```python
from build123d import *

# Parameters (mm, degrees)
BOSS_EXTRU_1_DEPTH       = 15
ESQUISSE6_W              = 100
ESQUISSE6_H              = 15
ENL_V_MAT_EXTRU_1_DEPTH  = 255
ENL_V_MAT_EXTRU_10_REACH = 393.106
ESQUISSE11_R             = 2.25
ENL_V_MAT_EXTRU_11_REACH = 393.106
ESQUISSE8_R              = 2.25
CONG_10_R                = 10
CONG_11_R                = 2
ENL_V_MAT_EXTRU_12_REACH = 391.991
ENL_V_MAT_EXTRU_13_REACH = 391.991
ESQUISSE13_W             = 20
ESQUISSE13_H             = 143.033455182
ESQUISSE13_H_2           = 181.308681646
CONG_12_R                = 10
ENL_V_MAT_EXTRU_14_REACH = 376.645
ESQUISSE14_R             = 1.6


with BuildPart() as part:
    # Esquisse1 → Boss.-Extru.1 (new body)
    with BuildSketch(Plane(origin=(0, 0, 0), x_dir=(1, 0, 0), z_dir=(0, 1, 0))):
        Polygon((-76.643189126, -51.401333399), (63.356810874, 43.598666601), (163.356810874, 43.598666601), (303.356810874, -51.401333399), (303.356810874, -151.401333399), (163.356810874, -246.401333399), (63.356810874, -246.401333399), (-76.643189126, -151.401333399), align=None)
    extrude(amount=BOSS_EXTRU_1_DEPTH)

    # Esquisse6 → Enlèv. mat.-Extru.1 (cut)
    with BuildSketch(Plane.XY.offset(246.401333399)):
        with Locations((113.356810874, 7.5)):
            Rectangle(ESQUISSE6_W, ESQUISSE6_H)
    extrude(amount=-ENL_V_MAT_EXTRU_1_DEPTH, mode=Mode.SUBTRACT)

    # Esquisse11 → Enlèv. mat.-Extru.10 (cut, up to next)
    with BuildSketch(Plane(origin=(0, 15, 0), x_dir=(1, 0, 0), z_dir=(0, 1, 0)), mode=Mode.PRIVATE) as enl_v_mat_extru_10_sk1:
        with Locations(Location((53.356810874, -129.901333399, 0), (0, 0, 270))):
            Circle(ESQUISSE11_R)
    enl_v_mat_extru_10_tool1 = extrude(enl_v_mat_extru_10_sk1.sketch, amount=-ENL_V_MAT_EXTRU_10_REACH, mode=Mode.PRIVATE) & part.part
    # Esquisse11 → Enlèv. mat.-Extru.10 (cut, up to next)
    with BuildSketch(Plane(origin=(0, 15, 0), x_dir=(1, 0, 0), z_dir=(0, 1, 0)), mode=Mode.PRIVATE) as enl_v_mat_extru_10_sk2:
        with Locations(Location((53.356810874, -184.901333399, 0), (0, 0, 270))):
            Circle(ESQUISSE11_R)
    enl_v_mat_extru_10_tool2 = extrude(enl_v_mat_extru_10_sk2.sketch, amount=-ENL_V_MAT_EXTRU_10_REACH, mode=Mode.PRIVATE) & part.part
    # Esquisse11 → Enlèv. mat.-Extru.10 (cut, up to next)
    with BuildSketch(Plane(origin=(0, 15, 0), x_dir=(1, 0, 0), z_dir=(0, 1, 0)), mode=Mode.PRIVATE) as enl_v_mat_extru_10_sk3:
        with Locations(Location((173.356810874, -129.901333399, 0), (0, 0, 270))):
            Circle(ESQUISSE11_R)
    enl_v_mat_extru_10_tool3 = extrude(enl_v_mat_extru_10_sk3.sketch, amount=-ENL_V_MAT_EXTRU_10_REACH, mode=Mode.PRIVATE) & part.part
    # Esquisse11 → Enlèv. mat.-Extru.10 (cut, up to next)
    with BuildSketch(Plane(origin=(0, 15, 0), x_dir=(1, 0, 0), z_dir=(0, 1, 0)), mode=Mode.PRIVATE) as enl_v_mat_extru_10_sk4:
        with Locations(Location((173.356810874, -184.901333399, 0), (0, 0, 270))):
            Circle(ESQUISSE11_R)
    enl_v_mat_extru_10_tool4 = extrude(enl_v_mat_extru_10_sk4.sketch, amount=-ENL_V_MAT_EXTRU_10_REACH, mode=Mode.PRIVATE) & part.part
    add(enl_v_mat_extru_10_tool1.solids().sort_by_distance((53.356811, 15, 129.901333))[0], mode=Mode.SUBTRACT)
    add(enl_v_mat_extru_10_tool2.solids().sort_by_distance((53.356811, 15, 184.901333))[0], mode=Mode.SUBTRACT)
    add(enl_v_mat_extru_10_tool3.solids().sort_by_distance((173.356811, 15, 129.901333))[0], mode=Mode.SUBTRACT)
    add(enl_v_mat_extru_10_tool4.solids().sort_by_distance((173.356811, 15, 184.901333))[0], mode=Mode.SUBTRACT)

    # Esquisse8 → Enlèv. mat.-Extru.11 (cut, up to next)
    with BuildSketch(Plane(origin=(0, 15, 0), x_dir=(1, 0, 0), z_dir=(0, 1, 0)), mode=Mode.PRIVATE) as enl_v_mat_extru_11_sk1:
        with Locations(Location((180.356810874, -120.901333399, 0), (0, 0, 270))):
            Circle(ESQUISSE8_R)
    enl_v_mat_extru_11_tool1 = extrude(enl_v_mat_extru_11_sk1.sketch, amount=-ENL_V_MAT_EXTRU_11_REACH, mode=Mode.PRIVATE) & part.part
    # Esquisse8 → Enlèv. mat.-Extru.11 (cut, up to next)
    with BuildSketch(Plane(origin=(0, 15, 0), x_dir=(1, 0, 0), z_dir=(0, 1, 0)), mode=Mode.PRIVATE) as enl_v_mat_extru_11_sk2:
        with Locations(Location((180.356810874, -81.901333399, 0), (0, 0, 270))):
            Circle(ESQUISSE8_R)
    enl_v_mat_extru_11_tool2 = extrude(enl_v_mat_extru_11_sk2.sketch, amount=-ENL_V_MAT_EXTRU_11_REACH, mode=Mode.PRIVATE) & part.part
    # Esquisse8 → Enlèv. mat.-Extru.11 (cut, up to next)
    with BuildSketch(Plane(origin=(0, 15, 0), x_dir=(1, 0, 0), z_dir=(0, 1, 0)), mode=Mode.PRIVATE) as enl_v_mat_extru_11_sk3:
        with Locations(Location((46.356810874, -120.901333399, 0), (0, 0, 270))):
            Circle(ESQUISSE8_R)
    enl_v_mat_extru_11_tool3 = extrude(enl_v_mat_extru_11_sk3.sketch, amount=-ENL_V_MAT_EXTRU_11_REACH, mode=Mode.PRIVATE) & part.part
    # Esquisse8 → Enlèv. mat.-Extru.11 (cut, up to next)
    with BuildSketch(Plane(origin=(0, 15, 0), x_dir=(1, 0, 0), z_dir=(0, 1, 0)), mode=Mode.PRIVATE) as enl_v_mat_extru_11_sk4:
        with Locations(Location((46.356810874, -81.901333399, 0), (0, 0, 270))):
            Circle(ESQUISSE8_R)
    enl_v_mat_extru_11_tool4 = extrude(enl_v_mat_extru_11_sk4.sketch, amount=-ENL_V_MAT_EXTRU_11_REACH, mode=Mode.PRIVATE) & part.part
    add(enl_v_mat_extru_11_tool1.solids().sort_by_distance((180.356811, 15, 120.901333))[0], mode=Mode.SUBTRACT)
    add(enl_v_mat_extru_11_tool2.solids().sort_by_distance((180.356811, 15, 81.901333))[0], mode=Mode.SUBTRACT)
    add(enl_v_mat_extru_11_tool3.solids().sort_by_distance((46.356811, 15, 120.901333))[0], mode=Mode.SUBTRACT)
    add(enl_v_mat_extru_11_tool4.solids().sort_by_distance((46.356811, 15, 81.901333))[0], mode=Mode.SUBTRACT)

    # Congé10
    cong_10_edges = [part.edges().sort_by_distance(p)[0] for p in [
        (-76.643189126, 7.5, 51.401333399),
        (63.356810874, 7.5, -43.598666601),
        (163.356810874, 7.5, -43.598666601),
        (303.356810874, 7.5, 51.401333399),
        (303.356810874, 7.5, 151.401333399),
        (-76.643189126, 7.5, 151.401333399),
        (63.356810874, 7.5, -8.598666601),
        (163.356810874, 7.5, -8.598666601),
    ]]
    fillet(cong_10_edges, radius=CONG_10_R)

    # Congé11
    cong_11_edges = [part.edges().sort_by_distance(p)[0] for p in [
        (163.356810874, 7.5, 246.401333399),
        (63.356810874, 7.5, 246.401333399),
    ]]
    fillet(cong_11_edges, radius=CONG_11_R)

    # Esquisse12 → Enlèv. mat.-Extru.12 (cut, up to next)
    with BuildSketch(Plane(origin=(0, 15, 0), x_dir=(1, 0, 0), z_dir=(0, 1, 0)), mode=Mode.PRIVATE) as enl_v_mat_extru_12_sk1:
        with BuildLine():
            Line((34.940182765, -48.918575783), (15.793326272, -80.935246354))
            ThreePointArc((15.793326272, -80.935246354), (14.39255048, -85.48771654), (15.256670784, -90.171780344))
            Line((15.256670784, -90.171780344), (27.943631129, -118.361875593))
            ThreePointArc((27.943631129, -118.361875593), (31.633138728, -122.655474578), (37.06267458, -124.257847507))
            Line((37.06267458, -124.257847507), (53.356810874, -124.257847507))
            ThreePointArc((53.356810874, -124.257847507), (57.183645198, -123.496642832), (60.427878686, -121.328915318))
            Line((60.427878686, -121.328915318), (63.356810874, -118.39998313))
            Line((63.356810874, -118.39998313), (63.356810874, -59.592280682))
            Line((63.356810874, -59.592280682), (64.824779414, -43.572926285))
            ThreePointArc((64.824779414, -43.572926285), (48.973323725, -41.163150472), (34.940182765, -48.918575783))
        make_face()
    enl_v_mat_extru_12_tool1 = extrude(enl_v_mat_extru_12_sk1.sketch, amount=-ENL_V_MAT_EXTRU_12_REACH, mode=Mode.PRIVATE) & part.part
    # Esquisse12 → Enlèv. mat.-Extru.12 (cut, up to next)
    with BuildSketch(Plane(origin=(0, 15, 0), x_dir=(1, 0, 0), z_dir=(0, 1, 0)), mode=Mode.PRIVATE) as enl_v_mat_extru_12_sk2:
        with BuildLine():
            Line((166.285743062, -121.328915318), (163.356810874, -118.39998313))
            Line((163.356810874, -118.39998313), (163.356810874, -73.642376596))
            Line((163.356810874, -73.642376596), (176.462200108, -67.250451181))
            ThreePointArc((176.462200108, -67.250451181), (187.921289626, -66.549583242), (196.519678004, -74.156794674))
            Line((196.519678004, -74.156794674), (206.924784537, -95.490424571))
            ThreePointArc((206.924784537, -95.490424571), (205.909865534, -114.856232791), (188.948903611, -124.257847507))
            Line((188.948903611, -124.257847507), (173.356810874, -124.257847507))
            ThreePointArc((173.356810874, -124.257847507), (169.529976551, -123.496642832), (166.285743062, -121.328915318))
        make_face()
    enl_v_mat_extru_12_tool2 = extrude(enl_v_mat_extru_12_sk2.sketch, amount=-ENL_V_MAT_EXTRU_12_REACH, mode=Mode.PRIVATE) & part.part
    add(enl_v_mat_extru_12_tool1.solids().sort_by_distance((43.224361, 15, 84.406415))[0], mode=Mode.SUBTRACT)
    add(enl_v_mat_extru_12_tool2.solids().sort_by_distance((183.873626, 15, 97.045657))[0], mode=Mode.SUBTRACT)

    # Esquisse13 → Enlèv. mat.-Extru.13 (cut, up to next)
    with BuildSketch(Plane(origin=(0, 15, 0), x_dir=(1, 0, 0), z_dir=(0, 1, 0)), mode=Mode.PRIVATE) as enl_v_mat_extru_13_sk1:
        with Locations((-66.643189126, -101.968599131)):
            Rectangle(ESQUISSE13_W, ESQUISSE13_H)
    enl_v_mat_extru_13_tool1 = extrude(enl_v_mat_extru_13_sk1.sketch, amount=-ENL_V_MAT_EXTRU_13_REACH, mode=Mode.PRIVATE) & part.part
    # Esquisse13 → Enlèv. mat.-Extru.13 (cut, up to next)
    with BuildSketch(Plane(origin=(0, 15, 0), x_dir=(1, 0, 0), z_dir=(0, 1, 0)), mode=Mode.PRIVATE) as enl_v_mat_extru_13_sk2:
        with Locations((293.356810874, -101.059068944)):
            Rectangle(ESQUISSE13_W, ESQUISSE13_H_2)
    enl_v_mat_extru_13_tool2 = extrude(enl_v_mat_extru_13_sk2.sketch, amount=-ENL_V_MAT_EXTRU_13_REACH, mode=Mode.PRIVATE) & part.part
    add(enl_v_mat_extru_13_tool1.solids().sort_by_distance((-66.643189, 15, 101.968599))[0], mode=Mode.SUBTRACT)
    add(enl_v_mat_extru_13_tool2.solids().sort_by_distance((293.356811, 15, 101.059069))[0], mode=Mode.SUBTRACT)

    # Congé12
    cong_12_edges = [part.edges().sort_by_distance(p)[0] for p in [
        (-56.643189126, 7.5, 37.829904828),
        (-56.643189126, 7.5, 164.97276197),
        (283.356810874, 7.5, 37.829904828),
        (283.356810874, 7.5, 164.97276197),
    ]]
    fillet(cong_12_edges, radius=CONG_12_R)

    # Esquisse14 → Enlèv. mat.-Extru.14 (cut, up to next)
    with BuildSketch(Plane(origin=(0, 15, 0), x_dir=(1, 0, 0), z_dir=(0, 1, 0)), mode=Mode.PRIVATE) as enl_v_mat_extru_14_sk1:
        with Locations(Location((-42.643189126, -51.403530316, 0), (0, 0, 270))):
            Circle(ESQUISSE14_R)
    enl_v_mat_extru_14_tool1 = extrude(enl_v_mat_extru_14_sk1.sketch, amount=-ENL_V_MAT_EXTRU_14_REACH, mode=Mode.PRIVATE) & part.part
    # Esquisse14 → Enlèv. mat.-Extru.14 (cut, up to next)
    with BuildSketch(Plane(origin=(0, 15, 0), x_dir=(1, 0, 0), z_dir=(0, 1, 0)), mode=Mode.PRIVATE) as enl_v_mat_extru_14_sk2:
        with Locations(Location((-42.643189126, -151.403530316, 0), (0, 0, 270))):
            Circle(ESQUISSE14_R)
    enl_v_mat_extru_14_tool2 = extrude(enl_v_mat_extru_14_sk2.sketch, amount=-ENL_V_MAT_EXTRU_14_REACH, mode=Mode.PRIVATE) & part.part
    # Esquisse14 → Enlèv. mat.-Extru.14 (cut, up to next)
    with BuildSketch(Plane(origin=(0, 15, 0), x_dir=(1, 0, 0), z_dir=(0, 1, 0)), mode=Mode.PRIVATE) as enl_v_mat_extru_14_sk3:
        with Locations(Location((73.359258963, 29.598666601, 0), (0, 0, 270))):
            Circle(ESQUISSE14_R)
    enl_v_mat_extru_14_tool3 = extrude(enl_v_mat_extru_14_sk3.sketch, amount=-ENL_V_MAT_EXTRU_14_REACH, mode=Mode.PRIVATE) & part.part
    # Esquisse14 → Enlèv. mat.-Extru.14 (cut, up to next)
    with BuildSketch(Plane(origin=(0, 15, 0), x_dir=(1, 0, 0), z_dir=(0, 1, 0)), mode=Mode.PRIVATE) as enl_v_mat_extru_14_sk4:
        with Locations(Location((153.359258963, 29.598666601, 0), (0, 0, 270))):
            Circle(ESQUISSE14_R)
    enl_v_mat_extru_14_tool4 = extrude(enl_v_mat_extru_14_sk4.sketch, amount=-ENL_V_MAT_EXTRU_14_REACH, mode=Mode.PRIVATE) & part.part
    # Esquisse14 → Enlèv. mat.-Extru.14 (cut, up to next)
    with BuildSketch(Plane(origin=(0, 15, 0), x_dir=(1, 0, 0), z_dir=(0, 1, 0)), mode=Mode.PRIVATE) as enl_v_mat_extru_14_sk5:
        with Locations(Location((269.356810874, -51.399136482, 0), (0, 0, 270))):
            Circle(ESQUISSE14_R)
    enl_v_mat_extru_14_tool5 = extrude(enl_v_mat_extru_14_sk5.sketch, amount=-ENL_V_MAT_EXTRU_14_REACH, mode=Mode.PRIVATE) & part.part
    # Esquisse14 → Enlèv. mat.-Extru.14 (cut, up to next)
    with BuildSketch(Plane(origin=(0, 15, 0), x_dir=(1, 0, 0), z_dir=(0, 1, 0)), mode=Mode.PRIVATE) as enl_v_mat_extru_14_sk6:
        with Locations(Location((269.356810874, -141.399136482, 0), (0, 0, 270))):
            Circle(ESQUISSE14_R)
    enl_v_mat_extru_14_tool6 = extrude(enl_v_mat_extru_14_sk6.sketch, amount=-ENL_V_MAT_EXTRU_14_REACH, mode=Mode.PRIVATE) & part.part
    add(enl_v_mat_extru_14_tool1.solids().sort_by_distance((-42.643189, 15, 51.40353))[0], mode=Mode.SUBTRACT)
    add(enl_v_mat_extru_14_tool2.solids().sort_by_distance((-42.643189, 15, 151.40353))[0], mode=Mode.SUBTRACT)
    add(enl_v_mat_extru_14_tool3.solids().sort_by_distance((73.359259, 15, -29.598667))[0], mode=Mode.SUBTRACT)
    add(enl_v_mat_extru_14_tool4.solids().sort_by_distance((153.359259, 15, -29.598667))[0], mode=Mode.SUBTRACT)
    add(enl_v_mat_extru_14_tool5.solids().sort_by_distance((269.356811, 15, 51.399136))[0], mode=Mode.SUBTRACT)
    add(enl_v_mat_extru_14_tool6.solids().sort_by_distance((269.356811, 15, 141.399136))[0], mode=Mode.SUBTRACT)


solid = part.part
```
Part model, mm, in its own coordinate system. A direction names the side the tool comes from. Give positions to 0.01 mm unless a question says otherwise; leave off trailing zeros. Order: outer loops, then holes, each group sorted by start corner. A loop starts at its lowest first (then second) coordinate and runs counter-clockwise, first axis right, second up. Notation, with made-up numbers: M 82.25,-9 L 103.25,-9 A16 cw 103.25,11 Z; hole C 17,14.5 d2. An arc over 180 degrees is marked long. Use a Markdown table: item, result. Add a question column.
(1) Saw through at B-B, the plane x = 42. Give the cut face in (y, z), and give its area (3 significant figures).
(2) Drop flat-ended pins along their axis: P1, Ø7.5, axis at y = 11, z = 25.5, coming from the -X side; P2, Ø4, axis at x = -7.5, y = 7.5, coming from the +Z side; P3, Ø7.5, axis at x = 110, y = 8, coming from the +Z side. Give the stop position or say it passes through.
(3) Saw through at D-D, the plane x = 84. Give the cut face in (y, z), and give its area (3 significant figures).
(4) Probe line 1 along X through (y, z) = (4.5, 141); line 2 along X through (y, z) = (3, 155.5); line 3 along X through (y, z) = (8.25, 131). List the from-to ranges inside material, lowest first. Write a range as [from, to].
(5) Mould opens along X. For faces 1 (the face through (191, 15, 131)), 2 (the face through (282.16, 7.4, 164.42)), 3 (the face through (163.357, 7, 181)) say: +X half, -X half, draft (parallel to the pull), parting line (faces both ways), or undercut.
(6) Saw through at C-C, the plane y = 6. Give the number of separate pieces and of enclosed holes in the cut face, and give its area (3 significant figures).
(7) Saw through at A-A, the plane z = 18. Give the cut face in (x, y).
(8) 3-axis set-ups, long thin cutter, end or side, ignore diameter. For faces 4 (the face through (160.35, 7.605, -5.747)), 5 (the face through (283.357, 8, 102)), 6 (the face through (169.8, 7.6, 70.5)): which of +Z, -Z, +X, -X, +Y, -Y reach the whole face in a straight line?
Answer key:
| question | item | result |
|---|---|---|
| 1 | outline | M 0,-29.11 L 15,-29.11 L 15,43.52 L 0,43.52 Z; M 0,124.26 L 15,124.26 L 15,231.91 L 0,231.91 Z |
| 1 | area | 2,700 mm^2 |
| 2 | P1 | x = -44 |
| 2 | P2 | z = 199.68 |
| 2 | P3 | z = -8.6 |
| 3 | outline | M 0,-43.6 L 15,-43.6 L 15,-8.6 L 0,-8.6 Z |
| 3 | area | 525 mm^2 |
| 4 | line 1 | [-56.64, 63.36], [163.36, 267.81], [270.91, 283.36] |
| 4 | line 2 | [-56.64, 63.36], [163.36, 283.36] |
| 4 | line 3 | [-56.64, 51.39], [55.32, 63.36], [163.36, 171.39], [175.32, 283.36] |
| 5 | face 1 | draft |
| 5 | face 2 | +X half |
| 5 | face 3 | undercut |
| 6 | separate pieces | 1 |
| 6 | enclosed holes | 10 |
| 6 | area | 48,100 mm^2 |
| 7 | outline | M -27.42,0 L 63.36,0 L 63.36,15 L -27.42,15 Z; M 163.36,0 L 254.13,0 L 254.13,15 L 163.36,15 Z |
| 8 | face 4 | +Z, +Y, -Y |
| 8 | face 5 | +Z, -Z, +X, +Y, -Y |
| 8 | face 6 | +Y, -Y |
